Input: dimensioned drawing with shaded views. Units: mm. Origin: part minimum x, y, z. Round coordinates to 2 decimals unless told otherwise and drop trailing zeros. Loops run counter-clockwise (first coordinate to the right, second up) from the corner with the lowest first, then second, coordinate; pieces in that order, holes last. Notation, with made-up numbers: (77.25, 89.25) - (124.25, 89.25) arc R25 ccw to (124.25, 110.25) - close; hole circle Ø11 at (89, 74). An arc over 180 degrees is marked (long way). Answer as CSV lines item,"result".
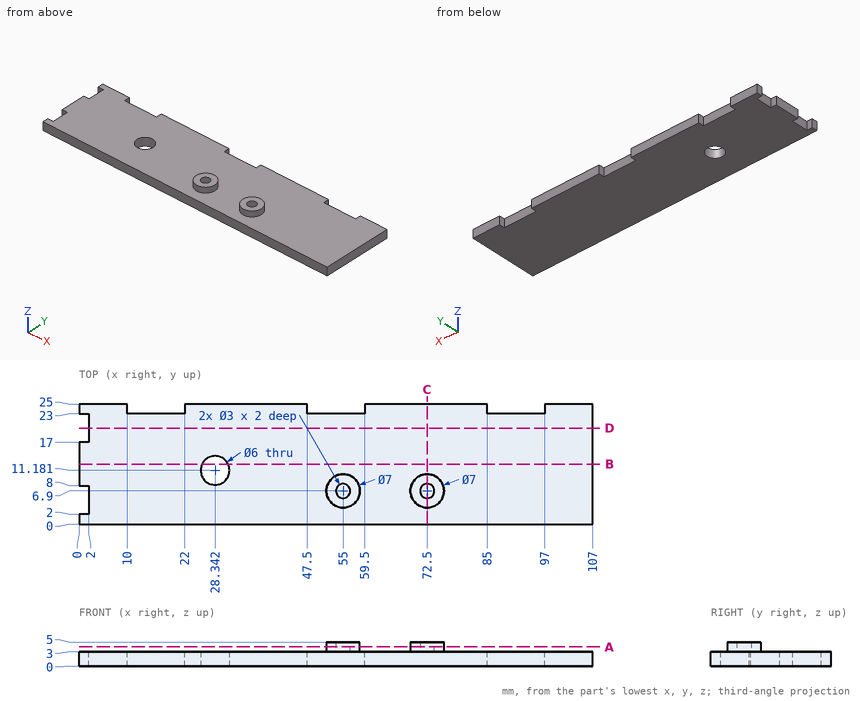
(1) Section B-B (y = 12.5). Output: boundary loops of the cut face in (x, z), and give its area (3 significant figures).
Findings below:
outline,"(0, 0) - (25.65, 0) - (25.65, 3) - (0, 3) - close; (31.04, 0) - (107, 0) - (107, 3) - (31.04, 3) - close"
area,"305 mm2"
(2) Section C-C (x = 72.5). Output: boundary loops of the cut face in (y, z).
Findings below:
outline,"(0, 0) - (25, 0) - (25, 3) - (10.4, 3) - (10.4, 5) - (8.4, 5) - (8.4, 3) - (5.4, 3) - (5.4, 5) - (3.4, 5) - (3.4, 3) - (0, 3) - close"
(3) Section A-A (z = 4). Output: boundary loops of the cut face in (x, y).
Findings below:
outline,"circle Ø7 at (55, 6.9); circle Ø7 at (72.5, 6.9); hole circle Ø3 at (55, 6.9); hole circle Ø3 at (72.5, 6.9)"
(4) Material intervals for line 1 along Y through (x, z) = (55, 4.45); line 2 along X through (y, z) = (23.25, 1.8); line 3 along X through (y, z) = (6.25, 4.5), sorted ascending.
Findings below:
line 1,"3.4 to 5.4, 8.4 to 10.4"
line 2,"0 to 10, 22 to 47.5, 59.5 to 85, 97 to 107"
line 3,"51.56 to 53.65, 56.35 to 58.44, 69.06 to 71.15, 73.85 to 75.94"
(5) Pin query (flat end, axial travel): P1, Ø1, axis at x = 92, z = 1, coming from the +Y side; P2, Ø6, axis at x = 12.5, y = 8.5, coming from the +Z side; P3, Ø0.9, axis at y = 6, z = 1.5, coming from the -X side. Return the tip coordinate at first contact, or that it passes through.
Findings below:
P1,"y = 23"
P2,"z = 3"
P3,"x = 2"
(6) Section D-D (y = 20). Output: boundary loops of the cut face in (x, z).
Findings below:
outline,"(2, 0) - (107, 0) - (107, 3) - (2, 3) - close"
